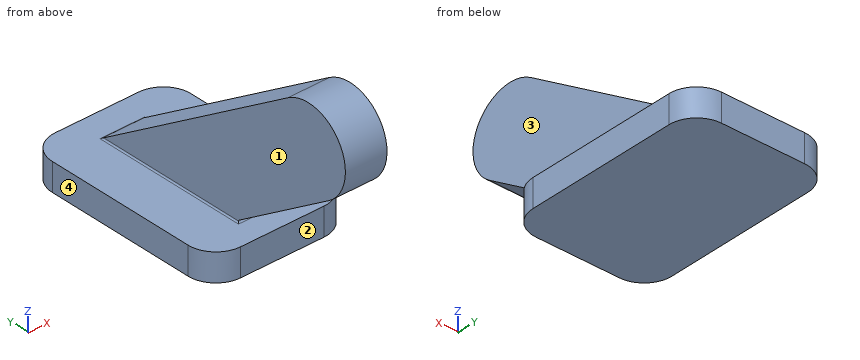
```python
from build123d import *

# Parameters (mm, degrees)
SKETCH1_W           = 10
SKETCH1_H           = 15
BOSS_EXTRUDE1_DEPTH = 2
BOSS_EXTRUDE2_DEPTH = 1.5
FILLET1_R           = 2
FILLET2_R           = 0.1


with BuildPart() as part:
    # Sketch1 → Boss-Extrude1 (new body)
    with BuildSketch(Plane.XY):
        Rectangle(SKETCH1_W, SKETCH1_H)
    extrude(amount=BOSS_EXTRUDE1_DEPTH)

    # Sketch3 → Boss-Extrude2 (add, symmetric)
    with BuildSketch(Plane(origin=(0, 0, 0), x_dir=(0, 0, -1), z_dir=(1, 0, 0))):
        with BuildLine():
            Line((-2, 5.427204202), (-12, -9.648363026))
            ThreePointArc((-12, -9.648363026), (-11.158312395, -13.806675422), (-7, -12.964987817))
            Line((-7, -12.964987817), (-2, -5.427204202))
            Line((-2, -5.427204202), (-2, 5.427204202))
        make_face()
    extrude(amount=BOSS_EXTRUDE2_DEPTH, both=True)

    # Fillet1
    fillet1_edges = [part.edges().sort_by_distance(p)[0] for p in [
        (5, -7.5, 1),
        (-5, -7.5, 1),
        (-5, 7.5, 1),
        (5, 7.5, 1),
    ]]
    fillet(fillet1_edges, radius=FILLET1_R)

    # Fillet2
    fillet2_edges = [part.edges().sort_by_distance(p)[0] for p in [
        (-1.5, 0, 2),
        (0, -5.427204202, 2),
        (0, 5.427204202, 2),
        (1.5, 0, 2),
    ]]
    fillet(fillet2_edges, radius=FILLET2_R)


solid = part.part
```
Geometry check sheet. Reference: the model listing, model coordinates, mm. Face numbers are marked on the shaded views. A direction names the side the tool comes from. Round coordinates to 2 decimals unless told otherwise and drop trailing zeros. Order: outer loops, then holes, each group sorted by start corner. A loop starts at its lowest first (then second) coordinate and runs counter-clockwise, first axis right, second up. Notation, with made-up numbers: (37, 21.25) - (61, 21.25) arc R25 cw to (61, 50.25) - close; hole circle Ø10 at (7, -30.75). An arc over 180 degrees is marked (long way). Use a Markdown table: item, result. Add a question column.
(1) Sectioned sample at D-D, the plane x = -2.5. Enter the section's corners in (y, z).
(2) Material ranges on line 1 along X through (y, z) = (-5.75, 6.25); line 2 along Z through (x, y) = (-4, -1); line 3 along Y through (x, z) = (1.25, 0.5), recorded low to high. Write a range as [from, to].
(3) Depth check by flat-ended pin: pin 1 (4 mm diameter, centred on x = 3, y = 2, fed in from +Z); pin 2 (5 mm diameter, centred on y = -7.5, z = 5.5, fed in from +X); pin 3 (1 mm diameter, centred on x = -1.5, y = 2.5, fed in from -Z); pin 4 (5 mm diameter, centred on x = 0.5, z = 7.5, fed in from +Y). Enter the tip coordinate at first touch or a pass-through.
(4) Tool access check on the marked faces 1, 2, 3 and 4. Record the directions out of +Z, -Z, +X, -X, +Y, -Y that give a thin tool (end or side, any length) a straight path to the whole face; none if there is none.
(5) Sectioned sample at A-A, the plane x = 1. Enter the section's corners in (y, z).
(6) Sectioned sample at C-C, the plane z = 10.5. Enter the section's corners in (x, y).
(7) Sectioned sample at B-B, the plane y = 2. Enter the section's corners in (x, z).
Answers below:
| question | item | result |
|---|---|---|
| 1 | outline | (-7.5, 0) - (7.5, 0) - (7.5, 2) - (-7.5, 2) - close |
| 2 | line 1 | [-1.5, 1.5] |
| 2 | line 2 | [0, 2] |
| 2 | line 3 | [-7.5, 7.5] |
| 3 | pin 1 | z = 5.15 |
| 3 | pin 2 | x = 1.5 |
| 3 | pin 3 | z = 0 |
| 3 | pin 4 | y = 0.9 |
| 4 | face 1 | +Z, -X, +Y, -Y |
| 4 | face 2 | -Z, +X, -X, -Y |
| 4 | face 3 | +Z, +X, +Y, -Y |
| 4 | face 4 | +Z, -Z, -X, +Y, -Y |
| 5 | outline | (-12.96, 7) - (-5.7, 2.18) arc R0.1 cw to (-5.76, 2) - (-7.5, 2) - (-7.5, 0) - (7.5, 0) - (7.5, 2) - (5.46, 2) arc R0.1 cw to (5.4, 2.02) - (-9.65, 12) arc R3 ccw to start |
| 6 | outline | (-1.5, -14.14) - (1.5, -14.14) - (1.5, -7.39) - (-1.5, -7.39) - close |
| 7 | outline | (-5, 0) - (5, 0) - (5, 2) - (1.6, 2) arc R0.1 cw to (1.5, 2.1) - (1.5, 4.27) - (-1.5, 4.27) - (-1.5, 2.1) arc R0.1 cw to (-1.6, 2) - (-5, 2) - close |
